The listing builds one solid part. Answer for the finished solid, in the listing's coordinates (mm). Give positions to 0.01 mm unless a question says otherwise; leave off trailing zeros. Loops run counter-clockwise (first coordinate to the right, second up) from the corner with the lowest first, then second, coordinate; pieces in that order, holes last. Notation, with made-up numbers: (-28, -39.75) - (-23, -39.75) arc R23 ccw to (-23, -2.75) - close; hole circle Ø3 at (-6, -24.5). An arc over 180 degrees is marked (long way). Answer as CSV lines item,"result". Start each with the question number.
1) A cutting plane is placed at A-A (x = 0). Determine the outline of the cut face in (y, z), and give its area (3 significant figures).
2) For a pull along X with two mould halves and no side action, classify faces 1 (the face through (-13.67, 73.95, -3.03)), 2 (the face through (0.66, 73.95, -14.985)) as pulls with the +X half, pulls with the -X half, needs draft (parallel to the pull), parting line crosses it, or undercut.
3) A cutting plane is placed at C-C (z = 0). Determine the outline of the cut face in (x, y).
4) Flat-ended cylindrical pins translate along their axes: pin 1 (4 mm diameter, centred on x = 11, y = 25.5, fed in from +Z); pin 2 (2 mm diameter, centred on y = 46.5, z = 11.5, fed in from +X); pin 3 (4 mm diameter, centred on y = 122, z = 10, fed in from +X). Find the tip coordinate at first contact, or state that the pin passes through.
5) Find the intervals of material crossed by line 1 along Z through (x, y) = (-3, 42.5); line 2 along X through (y, z) = (67, 0); line 3 along Z through (x, y) = (-12.5, 122), in increasing order.
6) A cutting plane is placed at D-D (y = 92). Determine the outline of the cut face in (x, z).
```python
from build123d import *

# Parameters (mm, degrees)
SKETCH1_R           = 15
SKETCH1_R_2         = 14
BOSS_EXTRUDE1_DEPTH = 150
SKETCH2_W           = 6
SKETCH2_H           = 6
CUT_EXTRUDE1_DEPTH  = 15


with BuildPart() as part:
    # Sketch1 → Boss-Extrude1 (new body)
    with BuildSketch(Plane(origin=(0, 0, 0), x_dir=(1, 0, 0), z_dir=(0, 1, 0))):
        with Locations(Location((0, 0, 0), (0, 0, 270))):
            Circle(SKETCH1_R)
        with Locations(Location((0, 0, 0), (0, 0, 270))):
            Circle(SKETCH1_R_2, mode=Mode.SUBTRACT)
    extrude(amount=BOSS_EXTRUDE1_DEPTH)

    # Sketch2 → Cut-Extrude1 (cut, symmetric)
    with BuildSketch(Plane(origin=(0, 0, 0), x_dir=(0, 0, -1), z_dir=(1, 0, 0))):
        with Locations((0, 130)):
            Rectangle(SKETCH2_W, SKETCH2_H)
        with Locations((0, 20)):
            Rectangle(SKETCH2_W, SKETCH2_H)
    extrude(amount=CUT_EXTRUDE1_DEPTH, both=True, mode=Mode.SUBTRACT)


solid = part.part
```
Ans:
1,outline,"(0, -15) - (150, -15) - (150, -14) - (0, -14) - close; (0, 14) - (150, 14) - (150, 15) - (0, 15) - close"
1,area,"300 mm2"
2,face 1,"undercut"
2,face 2,"parting line crosses it"
3,outline,"(-15, 0) - (-14, 0) - (-14, 17) - (-15, 17) - close; (-15, 23) - (-14, 23) - (-14, 127) - (-15, 127) - close; (-15, 133) - (-14, 133) - (-14, 150) - (-15, 150) - close; (14, 0) - (15, 0) - (15, 17) - (14, 17) - close; (14, 23) - (15, 23) - (15, 127) - (14, 127) - close; (14, 133) - (15, 133) - (15, 150) - (14, 150) - close"
4,pin 1,"z = 12"
4,pin 2,"x = 10.71"
4,pin 3,"x = 12.69"
5,line 1,"-14.7 to -13.67, 13.67 to 14.7"
5,line 2,"-15 to -14, 14 to 15"
5,line 3,"-8.29 to -6.3, 6.3 to 8.29"
6,outline,"circle Ø30 at (0, 0); hole circle Ø28 at (0, 0)"
